from build123d import *

# Parameters (mm, degrees)
BOSS_EXTRUDE1_DEPTH = 9.525


with BuildPart() as part:
    # Sketch1 → Boss-Extrude1 (new body)
    with BuildSketch(Plane(origin=(0, 0, 0), x_dir=(1, 0, 0), z_dir=(0, 1, 0))):
        with BuildLine():
            Line((-43.253160589, 22.606536767), (-34.672708234, 34.346684109))
            ThreePointArc((-34.672708234, 34.346684109), (-32.680204005, 35.559969312), (-30.413368559, 35.008978255))
            Line((-30.413368559, 35.008978255), (-6.614426983, 17.615185966))
            ThreePointArc((-6.614426983, 17.615185966), (-2.849545496, 15.578373329), (1.322663433, 14.621497696))
            ThreePointArc((1.322663433, 14.621497696), (13.956234084, -4.556441994), (-7.559797873, -12.585193267))
            ThreePointArc((-7.559797873, -12.585193267), (-11.492870345, -10.89585042), (-15.734319794, -10.31875))
            Line((-15.734319794, -10.31875), (-45.212, -10.31875))
            ThreePointArc((-45.212, -10.31875), (-47.367261469, -9.426011469), (-48.26, -7.27075))
            Line((-48.26, -7.27075), (-48.26, 7.27075))
            ThreePointArc((-48.26, 7.27075), (-47.367261469, 9.426011469), (-45.212, 10.31875))
            Line((-45.212, 10.31875), (-40.94192183, 10.31875))
            ThreePointArc((-40.94192183, 10.31875), (-38.044433785, 12.420775884), (-39.143399065, 15.82756691))
            Line((-39.143399065, 15.82756691), (-42.590866444, 18.347197092))
            ThreePointArc((-42.590866444, 18.347197092), (-43.804151646, 20.339701321), (-43.253160589, 22.606536767))
        make_face()
    extrude(amount=-BOSS_EXTRUDE1_DEPTH)


solid = part.part
Geometry: final body of the model. Coordinates: model frame, mm. A direction names the side the tool comes from. Give positions to 0.01 mm unless a question says otherwise; leave off trailing zeros. Loops run counter-clockwise (first coordinate to the right, second up) from the corner with the lowest first, then second, coordinate; pieces in that order, holes last. Notation, with made-up numbers: M 81,67 L 117,67 A26 ccw 117,86 Z; hole C 25,10.25 d11. An arc over 180 degrees is marked long. Put each result on its own line as item: value.
1) Cut plane B-B, the plane x = -25. Return the cut outline in (y, z) (3 decimals).
Computed values:
outline: M -9.525,-31.053 L 0,-31.053 L 0,10.319 L -9.525,10.319 Z
2) First-contact query: P1, Ø1, axis at x = -25, y = -1.5, coming from the +Z side; P2, Ø5, axis at y = -7, z = -10.5, coming from the -X side; P3, Ø3, axis at y = -2, z = -11.5, coming from the -X side. Flat tips, straight axial feed; report the tip coordinate or a pass-through.
Computed values:
P1: stops at z = 10.32
P2: stops at x = -48.17
P3: stops at x = -46.57
3) Mould query, pull axis Z, two halves, no side actions, for faces 4 (the flat face through (-43, -5, -10.319)), 5 (the cylindrical face through (-32.713, -4.696, -35.555)), 6 (the cylindrical face through (-47.343, -4.696, 9.45)). Classes: released by +Z, released by -Z, zero draft, split by the parting line, or undercut.
Computed values:
face 4: undercut
face 5: released by -Z
face 6: released by +Z
4) Cut plane C-C, the plane z = -27. Return the cut outline in (x, y) (3 decimals).
Computed values:
outline: M -40.042,-9.525 L -19.455,-9.525 L -19.455,0 L -40.042,0 Z
5) Reachability of faces 1 (the flat face through (-40.84, -4.7, -17.07)), 2 (the cylindrical face through (-2.91, -4.7, -15.6)), 3 (the flat face through (-30, -5, 10.319)) from +Z, -Z, +X, -X, +Y, -Y: full face, straight path, thin tool, end or side. Return the list, or none.
Computed values:
face 1: -X, +Y, -Y
face 2: -Z, +X, +Y, -Y
face 3: +Z, -X, +Y, -Y
6) Material intervals for L1, parallel to Z at x = -32, y = -8; L2, parallel to Z at x = -4, y = -2.25; L3, parallel to X at y = -1.5, z = -33, sorted ascending. Write a range as from..to.
Computed values:
L1: z = -35.59..10.32
L2: z = -16.06..14.13
L3: x = -35.66..-27.66
